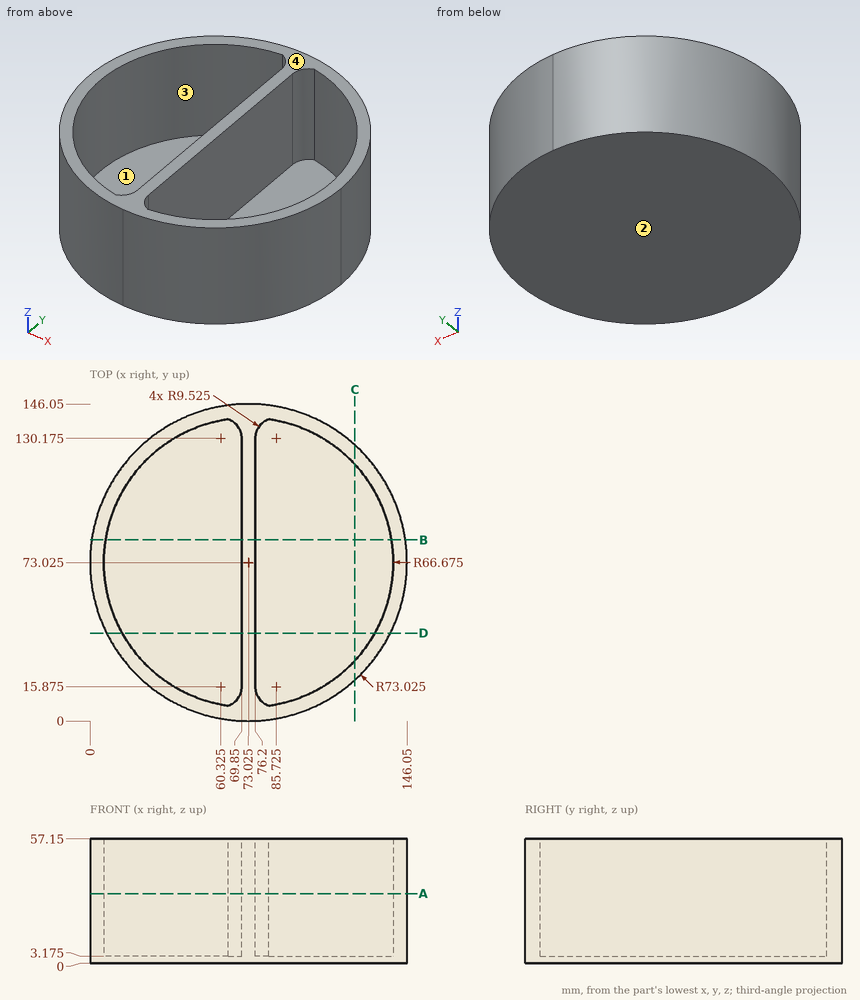
Check sheet for the drawn part. Datum: minimum x, y, z corner. Units: mm. A direction names the side the tool comes from. Round coordinates to 2 decimals unless told otherwise and drop trailing zeros. Loops run counter-clockwise (first coordinate to the right, second up) from the corner with the lowest first, then second, coordinate; pieces in that order, holes last.
Item 1: Mould release check, pull along Y, two halves, no side actions. Record for the marked faces 1 and 2: pulls with the +Y half, pulls with the -Y half, needs draft (parallel to the pull), parting line crosses it, or undercut.
Item 2: Cross-section at A-A on z = 32. Record the boundary of the cut face in (x, y) (3 decimals), then the cut area to 3 significant figures.
Item 3: Thickness scan on line 1 (X direction, y = 14.5, z = 30); line 2 (X direction, y = 63, z = 45); line 3 (Z direction, x = 104.5, y = 52) (3 decimals). Record the ranges inside material, lowest first.
Item 4: Cross-section at D-D on y = 40.5. Record the boundary of the cut face in (x, z) (3 decimals), then the cut area to 3 significant figures.
Item 5: Cross-section at C-C on x = 122. Record the boundary of the cut face in (y, z) (3 decimals), then the cut area to 3 significant figures.
Item 6: Cross-section at B-B on y = 83.5. Record the boundary of the cut face in (x, z) (3 decimals).
Item 7: Access from +Z, -Z, +X, -X, +Y, -Y to the whole of each face (thin tool, end or side, straight path). Record for the marked faces 3 and 4.
Item 8: Gauge pin test, flat ends, axial feed: pin 1 (12 mm diameter, centred on x = 101, y = 55.5, fed in from +Z) (3 decimals); pin 2 (5 mm diameter, centred on x = 21.5, z = 29, fed in from +Y); pin 3 (1 mm diameter, centred on x = 122, z = 49, fed in from +Y). Record the tip position at first contact, or that the pin passes through.
Answer sheet:
1. face 1: undercut
1. face 2: needs draft
2. outline: circle Ø146.05 at (73.025, 73.025); hole (63.771, 6.995) arc R9.525 ccw to (69.85, 15.875) - (69.85, 130.175) arc R9.525 ccw to (63.771, 139.055) arc R66.675 ccw to start; hole (76.2, 15.875) arc R9.525 ccw to (82.279, 6.995) arc R66.675 ccw to (82.279, 139.055) arc R9.525 ccw to (76.2, 130.175) - close
2. area: 3,700 mm2
3. line 1: x = 29.35 to 41.08, 69.75 to 76.3, 104.97 to 116.7
3. line 2: x = 0.69 to 7.11, 69.85 to 76.2, 138.94 to 145.36
3. line 3: z = 0 to 3.175
4. outline: (7.643, 0) - (138.407, 0) - (138.407, 57.15) - (131.229, 57.15) - (131.229, 3.175) - (76.2, 3.175) - (76.2, 57.15) - (69.85, 57.15) - (69.85, 3.175) - (14.821, 3.175) - (14.821, 57.15) - (7.643, 57.15) - close
4. area: 1,530 mm2
5. outline: (18.858, 0) - (127.192, 0) - (127.192, 57.15) - (118.269, 57.15) - (118.269, 3.175) - (27.781, 3.175) - (27.781, 57.15) - (18.858, 57.15) - close
5. area: 1,310 mm2
6. outline: (0.755, 0) - (145.295, 0) - (145.295, 57.15) - (138.872, 57.15) - (138.872, 3.175) - (76.2, 3.175) - (76.2, 57.15) - (69.85, 57.15) - (69.85, 3.175) - (7.178, 3.175) - (7.178, 57.15) - (0.755, 57.15) - close
7. face 3: +Z
7. face 4: +Z, +X, -X, +Y, -Y
8. pin 1: stops at z = 3.175
8. pin 2: stops at y = 127.15
8. pin 3: stops at y = 127.64
